from build123d import *

# Parameters (mm, degrees)
SKETCH1_W               = 92
SKETCH1_H               = 15
BOSS_EXTRUDE1_DEPTH     = 6
CUT_EXTRUDE1_DEPTH      = 54.227863457
CUT_EXTRUDE1_DEPTH_BACK = 54.227863457
SKETCH2_W               = 6.5
SKETCH2_H               = 5.5
CUT_EXTRUDE2_DEPTH      = 54.227863457
CUT_EXTRUDE2_DEPTH_BACK = 54.227863457
SKETCH3_W               = 6.5
SKETCH3_H               = 5.5
CUT_EXTRUDE3_DEPTH      = 54.227863457
CUT_EXTRUDE3_DEPTH_BACK = 54.227863457
SKETCH4_W               = 6.5
SKETCH4_H               = 5.5
CUT_EXTRUDE4_DEPTH      = 54.227863457
CUT_EXTRUDE4_DEPTH_BACK = 54.227863457
SKETCH5_W               = 6.5
SKETCH5_H               = 5.5
CUT_EXTRUDE5_DEPTH      = 54.227863457
CUT_EXTRUDE5_DEPTH_BACK = 4
SKETCH8_W               = 92
SKETCH8_H               = 11.3
SKETCH9_W               = 12
SKETCH9_H               = 7.5
CUT_EXTRUDE6_DEPTH      = 1.5
SKETCH10_W              = 12.5
SKETCH10_H              = 4
CUT_EXTRUDE7_DEPTH      = 1.5
CUT_EXTRUDE8_DEPTH      = 92
SKETCH13_W              = 0.5
SKETCH13_H              = 10
CUT_EXTRUDE9_DEPTH      = 0.6
FILLET1_R               = 0.25
FILLET2_R               = 0.25
SKETCH16_W              = 15
SKETCH16_H              = 0.5
BOSS_EXTRUDE2_DEPTH     = 0.75
FILLET3_R               = 0.5
FILLET4_R               = 0.25
SKETCH17_W              = 15
SKETCH17_H              = 0.5
BOSS_EXTRUDE3_DEPTH     = 0.75
FILLET5_R               = 0.5
FILLET6_R               = 0.25
LPATTERN1_COUNT         = 2
LPATTERN1_PITCH         = 47
LPATTERN2_COUNT         = 2
LPATTERN2_PITCH         = 47
FILLET7_R               = 0.5
FILLET8_R               = 0.25
FILLET9_R               = 0.5
FILLET10_R              = 0.25
CHAMFER1_SIZE           = 0.4
CHAMFER2_SIZE           = 0.4
CHAMFER3_SIZE           = 0.4
CHAMFER4_SIZE           = 0.4
CHAMFER5_SIZE           = 0.4


# Some blends are built 0.0001 mm under size
with BuildPart() as part:
    # Sketch1 → Boss-Extrude1 (new body)
    with BuildSketch(Plane.XY):
        with Locations((0.25, 18.154296875)):
            Rectangle(SKETCH1_W, SKETCH1_H)
    extrude(amount=BOSS_EXTRUDE1_DEPTH)

    # Sketch2 → Cut-Extrude1 (cut, two sides: drawn at the far end of the back side and taken through both)
    with BuildSketch(Plane.XY.offset(6).offset(-CUT_EXTRUDE1_DEPTH_BACK)):
        with Locations((-34.4, 18.154296875)):
            Rectangle(SKETCH2_W, SKETCH2_H)
    extrude(amount=CUT_EXTRUDE1_DEPTH + CUT_EXTRUDE1_DEPTH_BACK, mode=Mode.SUBTRACT)

    # Sketch3 → Cut-Extrude2 (cut, two sides: drawn at the far end of the back side and taken through both)
    with BuildSketch(Plane.XY.offset(6).offset(-CUT_EXTRUDE2_DEPTH_BACK)):
        with Locations((-11.35, 18.154296875)):
            Rectangle(SKETCH3_W, SKETCH3_H)
    extrude(amount=CUT_EXTRUDE2_DEPTH + CUT_EXTRUDE2_DEPTH_BACK, mode=Mode.SUBTRACT)

    # Sketch4 → Cut-Extrude3 (cut, two sides: drawn at the far end of the back side and taken through both)
    with BuildSketch(Plane.XY.offset(6).offset(-CUT_EXTRUDE3_DEPTH_BACK)):
        with Locations((11.7, 18.154296875)):
            Rectangle(SKETCH4_W, SKETCH4_H)
    extrude(amount=CUT_EXTRUDE3_DEPTH + CUT_EXTRUDE3_DEPTH_BACK, mode=Mode.SUBTRACT)

    # Sketch5 → Cut-Extrude4 (cut, two sides: drawn at the far end of the back side and taken through both)
    with BuildSketch(Plane.XY.offset(6).offset(-CUT_EXTRUDE4_DEPTH_BACK)):
        with Locations((34.75, 18.154296875)):
            Rectangle(SKETCH5_W, SKETCH5_H)
    extrude(amount=CUT_EXTRUDE4_DEPTH + CUT_EXTRUDE4_DEPTH_BACK, mode=Mode.SUBTRACT)

    # Sketch8 → Cut-Extrude5 (cut, two sides: drawn at the far end of the back side and taken through both)
    with BuildSketch(Plane.XY.offset(6).offset(-CUT_EXTRUDE5_DEPTH_BACK)):
        with Locations((0.25, 18.154296875)):
            Rectangle(SKETCH8_W, SKETCH8_H)
    extrude(amount=CUT_EXTRUDE5_DEPTH + CUT_EXTRUDE5_DEPTH_BACK, mode=Mode.SUBTRACT)

    # Sketch9 → Cut-Extrude6 (cut)
    with BuildSketch(Plane.XY.offset(2)):
        with Locations((34.25, 18.154296875)):
            Rectangle(SKETCH9_W, SKETCH9_H)
        with Locations((-33.9, 18.154296875)):
            Rectangle(SKETCH9_W, SKETCH9_H)
    extrude(amount=-CUT_EXTRUDE6_DEPTH, mode=Mode.SUBTRACT)

    # Sketch10 → Cut-Extrude7 (cut)
    with BuildSketch(Plane.XY.offset(2)):
        with Locations((11.7, 18.154296875)):
            Rectangle(SKETCH10_W, SKETCH10_H)
        with Locations((-11.35, 18.154296875)):
            Rectangle(SKETCH10_W, SKETCH10_H)
    extrude(amount=-CUT_EXTRUDE7_DEPTH, mode=Mode.SUBTRACT)

    # Sketch12 → Cut-Extrude8 (cut)
    with BuildSketch(Plane(origin=(46.25, 0, 0), x_dir=(0, 0, -1), z_dir=(1, 0, 0))):
        Polygon((-6, 25.654296875), (-6, 24.654296875), (-5, 25.654296875), align=None)
        Polygon((-6, 10.654296875), (-5, 10.654296875), (-6, 11.654296875), align=None)
    extrude(amount=-CUT_EXTRUDE8_DEPTH, mode=Mode.SUBTRACT)

    # Sketch13 → Cut-Extrude9 (cut)
    with BuildSketch(Plane(origin=(0, 0, 0), x_dir=(-1, 0, 0), z_dir=(0, 0, -1))):
        with Locations((43.5, 18.154296875)):
            Rectangle(SKETCH13_W, SKETCH13_H)
    extrude(amount=-CUT_EXTRUDE9_DEPTH, mode=Mode.SUBTRACT)

    # Fillet1
    fillet1_edges = [part.edges().sort_by_distance(p)[0] for p in [
        (-43.75, 18.154296875, 0),
    ]]
    fillet(fillet1_edges, radius=FILLET1_R)

    # Fillet2
    fillet2_edges = [part.edges().sort_by_distance(p)[0] for p in [
        (-43.25, 18.154296875, 0.6),
        (-43.5, 23.154296875, 0.6),
        (-43.75, 18.154296875, 0.6),
        (-43.5, 13.154296875, 0.6),
    ]]
    fillet(fillet2_edges, radius=FILLET2_R - 0.0001)  # a hair under: the kernel refuses the full size

    # Sketch16 → Boss-Extrude2 (add)
    with BuildSketch(Plane.XZ.offset(-23.804296875)):
        with Locations((-23.25, 4)):
            Rectangle(SKETCH16_W, SKETCH16_H)
    boss_extrude2 = extrude(amount=BOSS_EXTRUDE2_DEPTH)

    # Fillet3
    fillet3_edges = [part.edges().sort_by_distance(p)[0] for p in [
        (-23.25, 23.054296875, 4.25),
    ]]
    fillet(fillet3_edges, radius=FILLET3_R - 0.0001)  # a hair under: the kernel refuses the full size

    # Fillet4
    # the kernel refuses this fillet: 0.25 mm, written as the material it takes off along each edge
    with BuildSketch(Plane(origin=(-32.517583767, 23.054296875, 3.75), x_dir=(0, 0.707033489959235, 0.7071800648180521), z_dir=(1, 0, 0))) as fillet4_piece_1:
        with BuildLine():
            CenterArc((0.530239774, -0.176759657), FILLET4_R, 44.994478066, 179.999583566)
            Line((0.353444757, -0.35351803), (0.335765256, -0.371193867))
            Line((0.335765256, -0.371193867), (-0.017679502, -0.017675837))
            Line((-0.017679502, -0.017675837), (-0.017675837, 0.017679502))
            ThreePointArc((-0.017675837, 0.017679502), (-0.017605119, 0.017750205), (0.724712878, 0.017675966))
            Line((0.724712878, 0.017675966), (0.707033505, 0))
        make_face()
    extrude(amount=18.535167534, mode=Mode.SUBTRACT)

    # Sketch17 → Boss-Extrude3 (add)
    with BuildSketch(Plane(origin=(0, 12.504296875, 0), x_dir=(1, 0, 0), z_dir=(0, 1, 0))):
        with Locations((-23.25, -4)):
            Rectangle(SKETCH17_W, SKETCH17_H)
    boss_extrude3 = extrude(amount=BOSS_EXTRUDE3_DEPTH)

    # Fillet5
    fillet5_edges = [part.edges().sort_by_distance(p)[0] for p in [
        (-23.25, 13.254296875, 4.25),
    ]]
    fillet(fillet5_edges, radius=FILLET5_R - 0.0001)  # a hair under: the kernel refuses the full size

    # Fillet6
    # the kernel refuses this fillet: 0.25 mm, written as the material it takes off along each edge
    with BuildSketch(Plane(origin=(-13.982416233, 13.254296875, 3.75), x_dir=(0, -0.7070334915471351, 0.7071800632304811), z_dir=(-1, 0, 0))) as fillet6_piece_1:
        with BuildLine():
            CenterArc((0.530239775, -0.176759657), FILLET6_R, 44.994477938, 179.999583823)
            Line((0.353444759, -0.35351803), (0.335765257, -0.371193867))
            Line((0.335765257, -0.371193867), (-0.017679502, -0.017675837))
            Line((-0.017679502, -0.017675837), (-0.017675837, 0.017679502))
            ThreePointArc((-0.017675837, 0.017679502), (-0.017605119, 0.017750205), (0.72471288, 0.017675966))
            Line((0.72471288, 0.017675966), (0.707033507, 0))
        make_face()
    extrude(amount=18.535167534, mode=Mode.SUBTRACT)

    # LPattern1: Boss-Extrude3 ×2
    with Locations(*[(i * LPATTERN1_PITCH, 0, 0) for i in range(1, LPATTERN1_COUNT)]):
        add(boss_extrude3)

    # LPattern2: Boss-Extrude2 ×2
    with Locations(*[(i * LPATTERN2_PITCH, 0, 0) for i in range(1, LPATTERN2_COUNT)]):
        add(boss_extrude2)

    # Fillet7
    fillet7_edges = [part.edges().sort_by_distance(p)[0] for p in [
        (23.75, 23.054296875, 4.25),
    ]]
    fillet(fillet7_edges, radius=FILLET7_R - 0.0001)  # a hair under: the kernel refuses the full size

    # Fillet8
    # the kernel refuses this fillet: 0.25 mm, written as the material it takes off along each edge
    with BuildSketch(Plane(origin=(14.482416233, 23.054296875, 3.75), x_dir=(0, 0.707033489959235, 0.7071800648180521), z_dir=(1, 0, 0))) as fillet8_piece_1:
        with BuildLine():
            CenterArc((0.530239774, -0.176759657), FILLET8_R, 44.994478066, 179.999583566)
            Line((0.353444757, -0.35351803), (0.335765256, -0.371193867))
            Line((0.335765256, -0.371193867), (-0.017679502, -0.017675837))
            Line((-0.017679502, -0.017675837), (-0.017675837, 0.017679502))
            ThreePointArc((-0.017675837, 0.017679502), (-0.017605119, 0.017750205), (0.724712878, 0.017675966))
            Line((0.724712878, 0.017675966), (0.707033505, 0))
        make_face()
    extrude(amount=18.535167534, mode=Mode.SUBTRACT)

    # Fillet9
    fillet9_edges = [part.edges().sort_by_distance(p)[0] for p in [
        (23.75, 13.254296875, 4.25),
    ]]
    fillet(fillet9_edges, radius=FILLET9_R - 0.0001)  # a hair under: the kernel refuses the full size

    # Fillet10
    # the kernel refuses this fillet: 0.25 mm, written as the material it takes off along each edge
    with BuildSketch(Plane(origin=(33.017583767, 13.254296875, 3.75), x_dir=(0, -0.7070334947010828, 0.707180060077187), z_dir=(-1, 0, 0))) as fillet10_piece_1:
        with BuildLine():
            CenterArc((0.530239777, -0.176759656), FILLET10_R, 44.994477682, 179.999584334)
            Line((0.353444762, -0.35351803), (0.335765261, -0.371193867))
            Line((0.335765261, -0.371193867), (-0.017679502, -0.017675837))
            Line((-0.017679502, -0.017675837), (-0.017675837, 0.017679502))
            ThreePointArc((-0.017675837, 0.017679502), (-0.017605119, 0.017750205), (0.724712883, 0.017675966))
            Line((0.724712883, 0.017675966), (0.70703351, 0))
        make_face()
    extrude(amount=18.535167534, mode=Mode.SUBTRACT)

    # Chamfer1
    chamfer1_edges = [part.edges().sort_by_distance(p)[0] for p in [
        (0.25, 25.654296875, 0),
        (0.25, 10.654296875, 0),
    ]]
    chamfer(chamfer1_edges, length=CHAMFER1_SIZE)

    # Chamfer2
    chamfer2_edges = [part.edges().sort_by_distance(p)[0] for p in [
        (46.25, 18.154296875, 0),
        (-45.75, 18.154296875, 0),
    ]]
    chamfer(chamfer2_edges, length=CHAMFER2_SIZE)

    # Chamfer3
    chamfer3_edges = [part.edges().sort_by_distance(p)[0] for p in [
        (-45.75, 25.654296875, 2.7),
        (-45.75, 10.654296875, 2.7),
    ]]
    chamfer(chamfer3_edges, length=CHAMFER3_SIZE)

    # Chamfer4
    chamfer4_edges = [part.edges().sort_by_distance(p)[0] for p in [
        (-45.75, 11.354296875, 5.7),
        (-45.75, 24.954296875, 5.7),
    ]]
    chamfer(chamfer4_edges, length=CHAMFER4_SIZE)

    # Chamfer5
    chamfer5_edges = [part.edges().sort_by_distance(p)[0] for p in [
        (46.25, 24.229296875, 6),
        (46.25, 25.654296875, 2.7),
        (46.25, 10.654296875, 2.7),
        (46.25, 12.079296875, 6),
        (46.25, 25.154296875, 5.5),
        (46.25, 11.154296875, 5.5),
    ]]
    chamfer(chamfer5_edges, length=CHAMFER5_SIZE)


solid = part.part
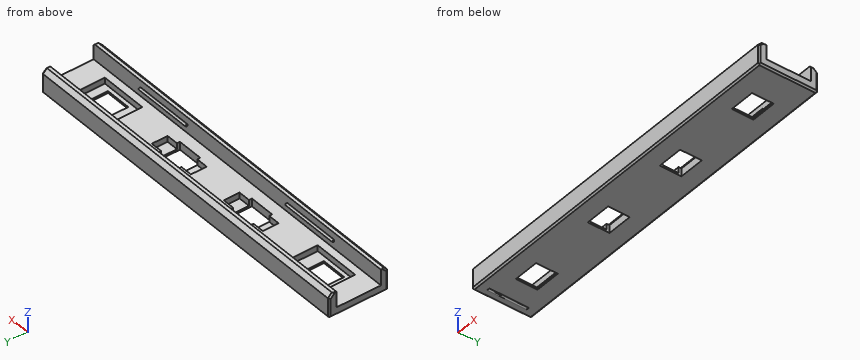
Part model, mm, in its own coordinate system. Give positions to 0.01 mm unless a question says otherwise; leave off trailing zeros. Loops run counter-clockwise (first coordinate to the right, second up) from the corner with the lowest first, then second, coordinate; pieces in that order, holes last.
(1) Band-saw the part on A-A (z = 3). Write the cut outline in (x, y).
Return value:
outline: (-45.75, 11.05) - (-45.35, 10.65) - (45.85, 10.65) - (46.25, 11.05) - (46.25, 12.5) - (-45.75, 12.5) - close; (-45.75, 23.8) - (46.25, 23.8) - (46.25, 25.25) - (45.85, 25.65) - (-45.35, 25.65) - (-45.75, 25.25) - close
(2) Band-saw the part on B-B (x = -35). Write the cut outline in (y, z).
Return value:
outline: (10.65, 0.4) - (11.05, 0) - (15.4, 0) - (15.4, 0.5) - (14.4, 0.5) - (14.4, 2) - (12.5, 2) - (12.5, 6) - (11.65, 6) - (10.65, 5) - close; (20.9, 0) - (25.25, 0) - (25.65, 0.4) - (25.65, 5) - (24.65, 6) - (23.8, 6) - (23.8, 2) - (21.9, 2) - (21.9, 0.5) - (20.9, 0.5) - close
(3) Drill centre lines: line 1 along X through (y, z) = (16.25, 1.5); line 2 along Y through (x, z) = (34.5, 4.5); line 3 along Z through (x, y) = (8, 23.5). Where is each one in solid material? Low to high.
Return value:
line 1: x = -45.75 to -39.9, -27.9 to -17.6, -5.1 to 5.45, 17.95 to 28.25, 40.25 to 46.25
line 2: y = 10.65 to 12.5, 23.8 to 25.65
line 3: z = 0 to 2
(4) Band-saw the part on D-D (y = 19). Count the separate pieces of the cut face and the enclosed holes in it, and give its area (3 significant figures).
Return value:
separate pieces: 5
enclosed holes: 0
area: 97.1 mm2
(5) Pin check, flat tip, straight feed: pin 1 (0.9 mm diameter, centred on x = 6.5, y = 18, fed in from +Z). Stop position of the tip, or through.
Return value:
pin 1: stops at z = 0.5
